CAD build for the part. Positions are in the model's coordinates, mm. A direction names the side the tool comes from. Round coordinates to 2 decimals unless told otherwise and drop trailing zeros. Write each loop counter-clockwise with the first axis right and the second up, starting at its lowest first coordinate (ties: lowest second). Pieces come first, ordered by that corner, then holes. Notation, with made-up numbers: M -32.5,50 L 8.5,50 A24 ccw 8.5,72 Z; hole C -2.75,-31 d2. An arc over 180 degrees is marked long. Write each question's results on one line, items separated by ' | '. Start each with the question number.
Autodesk Inventor part; units mm, degrees
ref_plane "YZ Plane" through (0, 0, 0) normal (1, 0, 0) x (0, 1, 0)
ref_plane "XZ Plane" through (0, 0, 0) normal (0, 1, 0) x (-1, 0, 0)
ref_plane "XY Plane" through (0, 0, 0) normal (0, 0, 1) x (1, 0, 0)
sketch "Esboço1" plane through (0, 0, 0) normal (0, 1, 0) x (-1, 0, 0)
  circle A0 centre (0, 0) radius 30.875
  dimension "d0" = 61.75
extrude "Extrusão1" add sketch "Esboço1" along normal blind 60.5
sketch "Esboço2" plane through (0, 60.5, 0) normal (0, 1, 0) x (1, 0, 0)
  line L0 (-28.4, -28.4) -> (28.4, -28.4)
  line L1 (28.4, -28.4) -> (28.4, 28.4)
  line L2 (28.4, 28.4) -> (-28.4, 28.4)
  line L3 (-28.4, 28.4) -> (-28.4, -28.4)
  point P0 (0, 0)
  dimension "d3" = 56.8
  dimension "d4" = 56.8
  dimension "d5" = 28.4
  dimension "d6" = 28.4
extrude "Extrusão2" add sketch "Esboço2" along normal blind 4.5
sketch "Esboço3" plane through (0, 65, 0) normal (0, 1, 0) x (1, 0, 0)
  line L0 (-28.4, -28.4) -> (28.4, -28.4)
  line L1 (28.4, -28.4) -> (28.4, 28.4)
  line L2 (-28.4, 28.4) -> (-28.4, -28.4)
  line L3 (28.4, 28.4) -> (-28.4, 28.4)
  point P0 (0, 0)
  point P1 (23.6, -23.6)
  point P2 (-23.6, -23.6)
  point P3 (-23.6, 23.6)
  point P4 (23.6, 23.6)
  dimension "d9" = 4.8
  dimension "d10" = 4.8
  dimension "d11" = 4.8
  dimension "d12" = 4.8
  dimension "d13" = 4.8
  dimension "d14" = 4.8
  dimension "d15" = 4.8
  dimension "d16" = 4.8
hole "Furo1" at (23.6, 65, 23.6) at (-23.6, 65, 23.6) at (-23.6, 65, -23.6) at (23.6, 65, -23.6) direction (0, -1, 0) diameter 5 depth 4.5
sketch "Esboço4" plane through (0, 65, 0) normal (0, 1, 0) x (1, 0, 0)
  circle A0 centre (0, 0) radius 3.25
  dimension "d24" = 6.5
extrude "Extrusão3" add sketch "Esboço4" along normal blind 18
sketch "Esboço5" plane through (0, 65, 0) normal (0, 1, 0) x (1, 0, 0)
  circle A0 centre (0, 0) radius 6
  circle A1 centre (0, 0) radius 3.25
  dimension "d27" = 12
extrude "Extrusão4" cut sketch "Esboço5" against normal blind 0.5
sketch "Esboço6" plane through (0, 0, 0) normal (0, 0, 1) x (1, 0, 0)
  line L0 (0, 0) -> (0, 60.5)
  line L1 (-12.1122, 60.5) -> (12.1122, 60.5)
  line L2 (0, 60.5) -> (-30.875, 60.5)
  line L3 (-30.875, 60.5) -> (-30.875, 52.5)
  line L4 (-30.875, 0) -> (-30.875, 60.5)
  arc A0 (-30.875, 34.25) -> (-30.875, 52.5) centre (-65.875, 43.375) ccw
  line L5 (30.875, 0) -> (-30.875, 0)
  line L6 (-30.875, 0) -> (-30.875, 8)
  arc A1 (-30.875, 8) -> (-30.875, 26.25) centre (-65.875, 17.125) ccw
  line L7 (-30.875, 26.25) -> (-30.875, 34.25)
  line L8 (-30.875, 0) -> (0, 0)
  line L9 (-30.875, 60.5) -> (-66.7077, 60.5)
  line L10 (-66.7077, 60.5) -> (-66.7077, 0)
  line L11 (-66.7077, 0) -> (-30.875, 0)
  dimension "d32" = 0
  dimension "d33" = 35
  dimension "d34" = 0
  dimension "d36" = 8
  dimension "d37" = 8
  dimension "d40" = 8
revolve "Revolução1" cut sketch "Esboço6" angle 360 about axis through (0, 0, 0) along (0, 1, 0) contours L11 L10 L9 L3 L4 | L4 A1 | A0 L4
equation "\"d4\" = d3"
equation "\"d22\" = Espessura"
equation "\"Raio_vergadura\" = Espessura"
equation "\"Largura_alívio_de_vergadura\" = Espessura"
equation "\"Profundidade_alívio_de_vergadura\" = 0.5 * Espessura"
equation "\"Tamanho_alívio_de_dobra\" = 4 * Espessura"
equation "\"Remanescente_mínimo\" = 2 * Espessura"
equation "\"Raiodetransição\" = Raio_vergadura"
equation "\"Tamanho_de_raio_de_Jacobi\" = Raio_vergadura"
equation "\"TamanhoFolga\" = Espessura"
properties part number "Motor" material "Steel"
1) Saw through at B-B, the plane z = 0. Write the cut outline in (x, y) (3 decimals).
2) 3-axis set-ups, long thin cutter, end or side, ignore diameter. For faces 1 (the face through (0, 63, 28.4)), 2 (the face through (-2.579, 73.88, 1.978)), 3 (the face through (0, 60.5, -29)), 4 (the face through (-25, 60.5, 26)): which of +Z, -Z, +X, -X, +Y, -Y reach the whole face in a straight line?
3) Drop flat-ended pins along their axis: pin 1 Ø8 at (x, z) = (-6.5, 23) entering from +Y; pin 2 Ø4 at (x, z) = (-23.6, 23.6) entering from +Y (3 decimals); pin 3 Ø1.3 at (y, z) = (62, 10) entering from -X; pin 4 Ø4 at (x, y) = (24.5, 38) entering from +Z. Give the stop position or say it passes through.
4) Saw through at A-A, the plane x = 0. Write the cut outline in (y, z) (3 decimals), plus the area to 3 significant figures.
5) Saw through at C-C, the plane x = -25. State how many separate pieces and enclosed holes the cut face has, plus the area to 3 significant figures.
6) Pull direction Z, two halves, no side cores. Call faces 5 (the face through (4.019, 3.944, -30.612)), 6 (the face through (26, 60.5, -22)), 7 (the face through (21.49, 62.72, -22.26)): pulls with the +Z half, pulls with the -Z half, needs draft (parallel to the pull), parting line crosses it, or undercut.
7) Wall check: line 1 along Z through (x, y) = (-23.6, 62.95); line 2 along X through (y, z) = (63, 23). Give the ranges that are in metal, low to high. Write a range as from..to.
Filled sheet:
1) outline: M -30.875,0 L 30.875,0 L 30.875,8 A36.17 cw 30.875,26.25 L 30.875,34.25 A36.17 cw 30.875,52.5 L 30.875,60.5 L 28.4,60.5 L 28.4,65 L 6,65 L 6,64.5 L 3.25,64.5 L 3.25,83 L -3.25,83 L -3.25,64.5 L -6,64.5 L -6,65 L -28.4,65 L -28.4,60.5 L -30.875,60.5 L -30.875,52.5 A36.17 cw -30.875,34.25 L -30.875,26.25 A36.17 cw -30.875,8 Z
2) face 1: +Z, +X, -X, +Y | face 2: +Y | face 3: -Z, +X, -X, +Y | face 4: +Z, -X, -Y
3) pin 1: stops at y = 65 | pin 2: passes through | pin 3: stops at x = -28.4 | pin 4: stops at z = 20.05
4) outline: M 0,-30.875 L 8,-30.875 A36.17 cw 26.25,-30.875 L 34.25,-30.875 A36.17 cw 52.5,-30.875 L 60.5,-30.875 L 60.5,-28.4 L 65,-28.4 L 65,-6 L 64.5,-6 L 64.5,-3.25 L 83,-3.25 L 83,3.25 L 64.5,3.25 L 64.5,6 L 65,6 L 65,28.4 L 60.5,28.4 L 60.5,30.875 L 52.5,30.875 A36.17 cw 34.25,30.875 L 26.25,30.875 A36.17 cw 8,30.875 L 0,30.875 Z | area: 4,050 mm^2
5) separate pieces: 3 | enclosed holes: 0 | area: 2,310 mm^2
6) face 5: parting line crosses it | face 6: needs draft | face 7: undercut
7) line 1: z = -28.4..-26.1, -21.1..21.1, 26.1..28.4 | line 2: x = -28.4..-26.03, -21.17..21.17, 26.03..28.4
